The model under review builds one solid part; all positions refer to its coordinate system, in mm. Face numbers are marked on the shaded views. A direction names the side the tool comes from. Round coordinates to 2 decimals unless told otherwise and drop trailing zeros. Order: outer loops, then holes, each group sorted by start corner. A loop starts at its lowest first (then second) coordinate and runs counter-clockwise, first axis right, second up.
Autodesk Inventor part; units mm, degrees
ref_plane "YZ Plane" through (0, 0, 0) normal (1, 0, 0) x (0, 1, 0)
ref_plane "XZ Plane" through (0, 0, 0) normal (0, 1, 0) x (-1, 0, 0)
ref_plane "XY Plane" through (0, 0, 0) normal (0, 0, 1) x (1, 0, 0)
sketch "Sketch1" plane through (0, 0, 0) normal (0, 0, 1) x (1, 0, 0)
  line L0 (-50.8, -25.4) -> (50.8, -25.4)
  line L1 (50.8, -25.4) -> (50.8, 25.4)
  line L2 (50.8, 25.4) -> (-50.8, 25.4)
  line L3 (-50.8, 25.4) -> (-50.8, -25.4)
  point P0 (0, 0)
  point P1 (0, 25.4)
  point P2 (50.8, 0)
  dimension "d10" = 6.5
  dimension "d0" = 50.8
  dimension "d2" = 101.6
extrude "Extrusion1" add sketch "Sketch1" along normal blind 15
sketch "Sketch2" plane through (0, 0, 15) normal (0, 0, 1) x (1, 0, 0)
  line L0 (50.8, -25.4) -> (50.8, 25.4)
  line L1 (50.8, 25.4) -> (-50.8, 25.4)
  line L2 (-45.339, 21.9075) -> (45.339, 21.9075)
  line L3 (45.339, 21.9075) -> (45.339, -21.9075)
  line L4 (45.339, -21.9075) -> (-45.339, -21.9075)
  line L5 (-45.339, -21.9075) -> (-45.339, 21.9075)
  point P0 (45.339, 0)
  point P1 (50.8, 0)
  point P2 (0, 21.9075)
  point P3 (0, 25.4)
  dimension "d5" = 43.815
  dimension "d7" = 90.678
hole "Hole1" at (-45.339, 21.9075, 15) at (45.339, 21.9075, 15) at (45.339, -21.9075, 15) at (-45.339, -21.9075, 15) direction (0, 0, -1) diameter 3.4 end through all
sketch "Sketch3" plane through (-50.8, -25.4, 0) normal (-1, 0, 0) x (0, 0, 1)
  line L0 (0, 50.8) -> (0, 0)
  line L1 (0, 0) -> (15, 0)
  circle A0 centre (6, 14.9) radius 5
  point P0 (0, 25.4)
  dimension "d15" = 6
  dimension "d16" = 14.9
  dimension "d17" = 10
extrude "Extrusion2" add sketch "Sketch3" along normal blind 10
sketch "Sketch4" plane through (-50.8, 25.4, 0) normal (-1, 0, 0) x (0, 0, 1)
  circle A0 centre (6, -35.9) radius 5
  line L0 (0, 0) -> (15, 0)
  line L1 (-3.5, -12.5) -> (11.5, -12.5)
  line L2 (11.5, -12.5) -> (11.5, -27.5)
  line L3 (11.5, -27.5) -> (-3.5, -27.5)
  line L4 (-3.5, -27.5) -> (-3.5, -12.5)
  point P0 (0, -27.9)
  point P1 (15, -31.5411)
  point P2 (0, -25.4)
  point P3 (-3.5, -20)
  point P4 (4, -12.5)
  dimension "d20" = 20
  dimension "d21" = 15
  dimension "d22" = 15
  dimension "d23" = 2
extrude "Extrusion3" add sketch "Sketch4" along normal blind 10 contours L1 L2 L3 L4
properties part number "electronics"
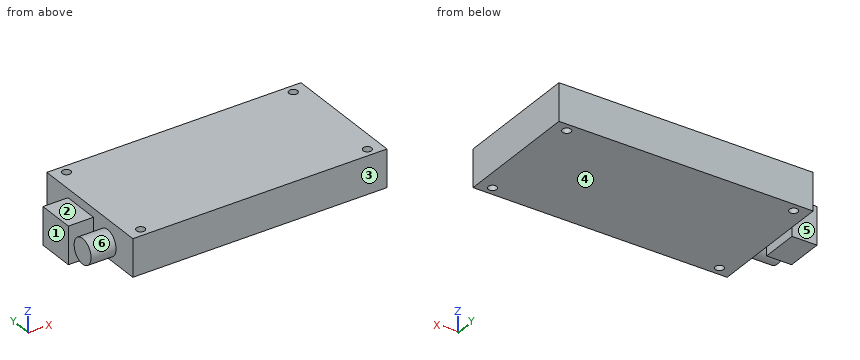
(1) To check wall thickness, follow probe 1 along X at (y, z) = (-20.5, 11); probe 2 along X at (y, z) = (21, 1.5); probe 3 along X at (y, z) = (-6, 1). State the ranges of each line that lie inside material, in increasing order.
Data:
probe 1: x = -50.8 to -46.29, -44.39 to 44.39, 46.29 to 50.8
probe 2: x = -50.8 to -46.78, -43.9 to 43.9, 46.78 to 50.8
probe 3: x = -50.8 to 50.8
(2) Consider section D-D (z = 12.5). Write out the cut boundary in (x, y), and give its area (3 significant figures).
Data:
outline: (-50.8, -25.4) - (50.8, -25.4) - (50.8, 25.4) - (-50.8, 25.4) - close; hole circle Ø3.4 at (-45.34, -21.91); hole circle Ø3.4 at (-45.34, 21.91); hole circle Ø3.4 at (45.34, -21.91); hole circle Ø3.4 at (45.34, 21.91)
area: 5,120 mm2
(3) Draft analysis for pull direction Y (two halves, no side actions). For the marked faces 3, 4, 5 and 6, state which applies: pulls with the +Y half, pulls with the -Y half, needs draft (parallel to the pull), parting line crosses it, or undercut.
Data:
face 3: pulls with the -Y half
face 4: needs draft
face 5: pulls with the +Y half
face 6: undercut
(4) For the marked faces 1 and 2, list the 3-axis set-ups (+Z, -Z, +X, -X, +Y, -Y) from which the entire face can be reached by the end or side of a thin tool; tool diameter is ignored.
Data:
face 1: +Z, -Z, -X, +Y, -Y
face 2: +Z, -X, +Y, -Y
(5) Insertion check: pin 1 (6 mm diameter, centred on x = -16, y = 19, fed in from -Z); pin 2 (5 mm diameter, centred on x = -58, z = 4.5, fed in from -Y); pin 3 (3 mm diameter, centred on x = 45.34, y = -21.91, fed in from -Z); pin 4 (3 mm diameter, centred on y = 5.5, z = -2, fed in from +X). Each pin has a flat end and moves straight along its axis. Give the tip position at first contact, or say it passes through.
Data:
pin 1: stops at z = 0
pin 2: stops at y = -15.5
pin 3: passes through
pin 4: stops at x = -50.8
(6) Consider section C-C (x = 14.5). Write out the cut boundary in (y, z), and give its area (3 significant figures).
Data:
outline: (-25.4, 0) - (25.4, 0) - (25.4, 15) - (-25.4, 15) - close
area: 762 mm2
(7) Consider section A-A (y = -10.5). Write out the cut boundary in (x, z), and give its area (3 significant figures).
Data:
outline: (-60.8, 1) - (-50.8, 1) - (-50.8, 0) - (50.8, 0) - (50.8, 15) - (-50.8, 15) - (-50.8, 11) - (-60.8, 11) - close
area: 1,620 mm2
(8) Consider section B-B (z = 2.5). Write out the cut boundary in (x, y).
Data:
outline: (-60.8, -14.07) - (-50.8, -14.07) - (-50.8, -25.4) - (50.8, -25.4) - (50.8, 25.4) - (-50.8, 25.4) - (-50.8, 12.9) - (-60.8, 12.9) - (-60.8, -2.1) - (-50.8, -2.1) - (-50.8, -6.93) - (-60.8, -6.93) - close; hole circle Ø3.4 at (-45.34, -21.91); hole circle Ø3.4 at (-45.34, 21.91); hole circle Ø3.4 at (45.34, -21.91); hole circle Ø3.4 at (45.34, 21.91)
